Input: dimensioned drawing with shaded views. Units: mm. Origin: part minimum x, y, z. Round coordinates to 2 decimals unless told otherwise and drop trailing zeros. Loops run counter-clockwise (first coordinate to the right, second up) from the corner with the lowest first, then second, coordinate; pieces in that order, holes last.
1) Section A-A, the plane y = 24. Return loops of the section in (x, z), and give its area (3 significant figures).
2) Section C-C, the plane x = 5.5. Return loops of the section in (y, z), and give its area (3 significant figures).
3) Draft query along Y for the marked faces 1, 2 and 3. Return one class per face: pulls with the +Y half, pulls with the -Y half, needs draft (parallel to the pull), parting line crosses it, or undercut.
4) Section B-B, the plane z = 14.4. Return loops of the section in (x, y).
5) Ray query, line 1 along Y through (x, z) = (5.25, 14.4); line 2 along Y through (x, z) = (2.5, 12.75) (1 decimal); line 3 along Y through (x, z) = (1.5, 19). Return the intervals inside material, ascending.
6) First-contact query: pin 1 (2 mm diameter, centred on x = 3.5, z = 21.5, fed in from -Y). Flat tip, straight axial feed; report the tip coordinate or a pass-through.
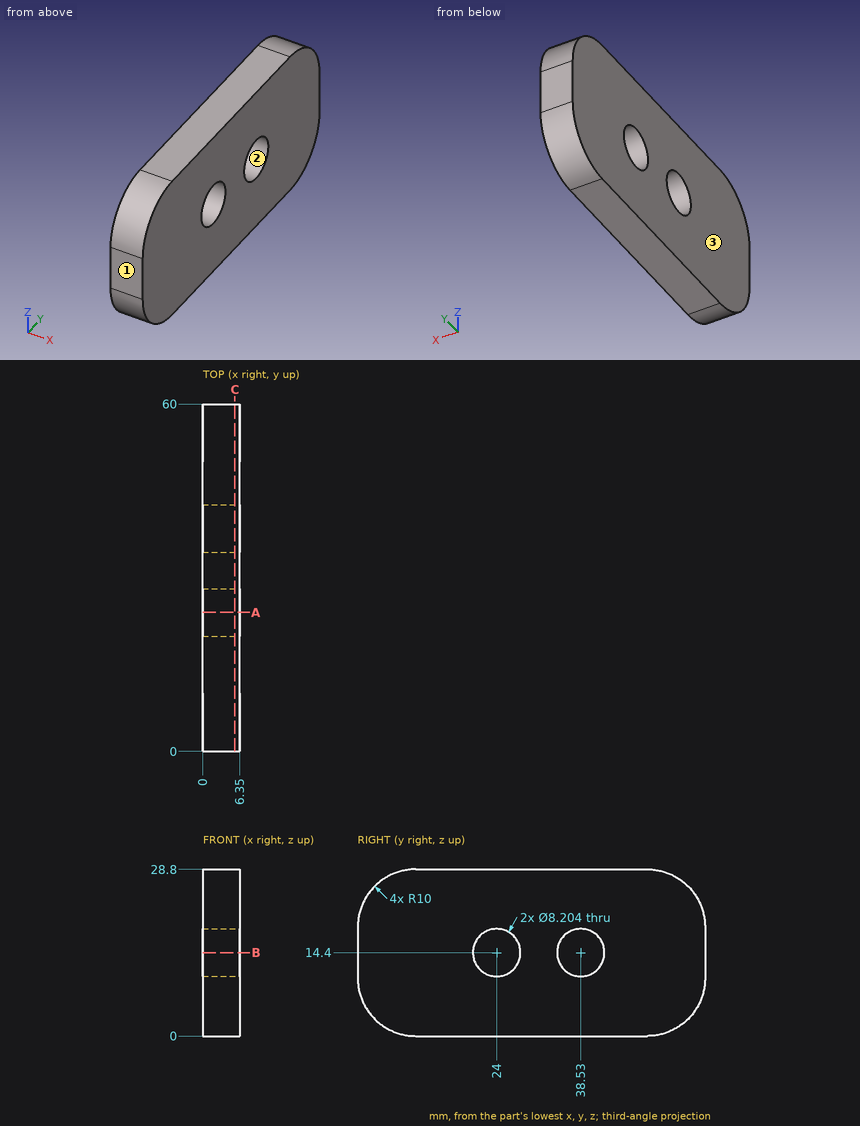
Final values:
1. outline: (0, 0) - (6.35, 0) - (6.35, 10.3) - (0, 10.3) - close; (0, 18.5) - (6.35, 18.5) - (6.35, 28.8) - (0, 28.8) - close
1. area: 131 mm2
2. outline: (0, 10) arc R10 ccw to (10, 0) - (50, 0) arc R10 ccw to (60, 10) - (60, 18.8) arc R10 ccw to (50, 28.8) - (10, 28.8) arc R10 ccw to (0, 18.8) - close; hole circle Ø8.2 at (24, 14.4); hole circle Ø8.2 at (38.53, 14.4)
2. area: 1,540 mm2
3. face 1: pulls with the -Y half
3. face 2: undercut
3. face 3: needs draft
4. outline: (0, 0) - (6.35, 0) - (6.35, 19.9) - (0, 19.9) - close; (0, 28.1) - (6.35, 28.1) - (6.35, 34.43) - (0, 34.43) - close; (0, 42.63) - (6.35, 42.63) - (6.35, 60) - (0, 60) - close
5. line 1: y = 0 to 19.9, 28.1 to 34.43, 42.63 to 60
5. line 2: y = 0 to 20.2, 27.8 to 34.8, 42.3 to 60
5. line 3: y = 0 to 60
6. pin 1: stops at y = 0.15
